The listing builds one solid part. Answer for the finished solid, in the listing's coordinates (mm). A direction names the side the tool comes from. Coordinates: 2 decimals unless noted, no trailing zeros. Loops run counter-clockwise (first coordinate to the right, second up) from the corner with the lowest first, then second, coordinate; pieces in that order, holes last. Notation, with made-up numbers: (78.25, 30) - (92.25, 30) arc R27 ccw to (92.25, 64) - close; hole circle Ø3 at (12, 0). An arc over 180 degrees is marked (long way). Return JSON: item names as keys, results as strings. Group by question number.
1. The mould has two halves that part along X. Classify faces 1 (the face through (-29.219, 17.594, 3.944)), 2 (the face through (11, 0, 8)): pulls with the +X half, pulls with the -X half, needs draft (parallel to the pull), parting line crosses it, or undercut.
2. Each of these flat-tipped pins is pushed along its axis until it touches: P1, Ø4, axis at y = -17.5, z = 4.5, coming from the -X side; P2, Ø4, axis at y = 19.5, z = 4, coming from the -X side; P3, Ø4, axis at x = 48, y = -18, coming from the +Z side; P4, Ø1.5, axis at x = 51, z = 1.5, coming from the +Y side. Where does it stop, or does it pass through?
3. Which of the six approach directions +Z, -Z, +X, -X, +Y, -Y give full straight-line access (tool end or side, diameter ignored) to faces 3 (the face through (40.757, 26.456, 3.944)), 4 (the face through (10, -29, 4))?
4. Find the intervals of material crossed by line 1 along Y through (x, z) = (10.75, 6); line 2 along X through (y, z) = (0.5, 2.5); line 3 along X through (y, z) = (-21.5, 1.25), in increasing order.
5. Section B-B (y = 1) is taken. Write down the section's boundary in (x, z), and give its area (3 significant figures).
6. Section A-A (x = -1) is taken. Write down the section's boundary in (y, z).
7. Section C-C (z = 3) is taken. State how many separate pieces and enclosed holes the cut face has, and give its area (3 significant figures).
8. Section D-D (x = 55) is taken. Write down the section's boundary in (y, z).
```python
from build123d import *

# Parameters (mm, degrees)
F0_R     = 1.6
F1_DEPTH = 8


with BuildPart() as f1:
    # F0 (on Top) → F1 (new body)
    with BuildSketch(Plane.XY):
        with BuildLine():
            ThreePointArc((7.75, 8.769357237), (9.5785114413, 4.5384947039), (10.2033247314, -0.028042301))
            ThreePointArc((10.2033247314, -0.028042301), (9.5785114413, -4.5945793059), (7.75, -8.825441839))
            Line((7.75, -8.825441839), (7.75, -18.0000000146))
            ThreePointArc((7.75, -18.0000000146), (10.7499999927, -15), (13.75, -18))
            Line((13.75, -18), (13.75, -8.8741196746))
            ThreePointArc((13.75, -8.8741196746), (11.25, 0), (13.75, 8.8741196746))
            Line((13.75, 8.8741196746), (13.75, 18))
            ThreePointArc((13.75, 18), (10.75, 15), (7.75, 18))
            Line((7.75, 18), (7.75, 8.769357237))
        make_face()
        with BuildLine():
            Line((7.75, 27.5), (7.75, 18))
            ThreePointArc((7.75, 18), (10.75, 21), (13.75, 18))
            Line((13.75, 18), (13.75, 27.5))
            Line((13.75, 27.5), (7.75, 27.5))
        make_face()
        with BuildLine():
            ThreePointArc((13.75, 18), (10.75, 21), (7.75, 18))
            ThreePointArc((7.75, 18), (10.75, 15), (13.75, 18))
        make_face()
        with Locations((10.75, 18)):
            Circle(F0_R, mode=Mode.SUBTRACT)
        with BuildLine():
            ThreePointArc((13.75, -18), (10.7499999927, -15), (7.75, -18.0000000146))
            ThreePointArc((7.75, -18.0000000146), (10.7500000073, -21), (13.75, -18))
        make_face()
        with Locations((10.75, -18)):
            Circle(F0_R, mode=Mode.SUBTRACT)
        with BuildLine():
            ThreePointArc((13.75, -18), (10.7500000073, -21), (7.75, -18.0000000146))
            Line((7.75, -18.0000000146), (7.75, -27.5))
            Line((7.75, -27.5), (13.75, -27.5))
            Line((13.75, -27.5), (13.75, -18))
        make_face()
        with BuildLine():
            ThreePointArc((-25.2919277241, 23.9346233209), (-18.7517090297, 26.593722392), (-11.75, 27.5))
            Line((-11.75, 27.5), (-11.75, 29))
            ThreePointArc((-11.75, 29), (-40.75, 0), (-11.75, -29))
            Line((-11.75, -29), (-11.75, -27.5))
            ThreePointArc((-11.75, -27.5), (-19.1538130954, -26.4845908341), (-26.0108698504, -23.5133492108))
            ThreePointArc((-26.0108698504, -23.5133492108), (-27.4397291664, -22.5850038451), (-28.8083510414, -21.5699480701))
            ThreePointArc((-28.8083510414, -21.5699480701), (-29.7732335043, -20.7704851664), (-30.7006958236, -19.9278982284))
            ThreePointArc((-30.7006958236, -19.9278982284), (-39.2465788178, -0.4337664292), (-31.3198462511, 19.3202256122))
            ThreePointArc((-31.3198462511, 19.3202256122), (-30.0815714824, 20.4988655048), (-28.77245464, 21.5982878495))
            ThreePointArc((-28.77245464, 21.5982878495), (-27.0767734107, 22.8328714098), (-25.2919277241, 23.9346233209))
        make_face()
        Polygon((-11.75, 29), (-11.75, 27.5), (7.75, 27.5), (13.75, 27.5), (33.25, 27.5), (33.25, 29), align=None)
        Polygon((7.75, -27.5), (-11.75, -27.5), (-11.75, -29), (33.25, -29), (33.25, -27.5), (13.75, -27.5), align=None)
        with BuildLine():
            Line((-23.9181566023, 16.8211807336), (-22.9196159905, 15.8385184773))
            ThreePointArc((-22.9196159905, 15.8385184773), (-22.2394609196, 16.8255111811), (-22, 18))
            ThreePointArc((-22, 18), (-22.2419209631, 19.180254221), (-22.9286666841, 20.1701562834))
            ThreePointArc((-22.9286666841, 20.1701562834), (-25.0876469222, 20.9987193962), (-27.1945482113, 20.0454725978))
            Line((-27.1945482113, 20.0454725978), (-26.1960075994, 19.0628103416))
            ThreePointArc((-26.1960075994, 19.0628103416), (-24.4314985308, 19.4955955601), (-23.4, 18))
            ThreePointArc((-23.4, 18), (-23.5352560913, 17.3561636218), (-23.9181566023, 16.8211807336))
        make_face()
        with BuildLine():
            ThreePointArc((-27.0590321397, 15.818168969), (-24.9852520778, 15.0000362504), (-22.9196159905, 15.8385184773))
            Line((-22.9196159905, 15.8385184773), (-23.9181566023, 16.8211807336))
            ThreePointArc((-23.9181566023, 16.8211807336), (-26.122267433, 16.8595984002), (-26.1960075994, 19.0628103416))
            Line((-26.1960075994, 19.0628103416), (-27.1945482113, 20.0454725978))
            ThreePointArc((-27.1945482113, 20.0454725978), (-27.9984596784, 17.9038773857), (-27.0590321397, 15.818168969))
        make_face()
        with BuildLine():
            Line((-22.9286666841, 20.1701562834), (-25.2919277241, 23.9346233209))
            ThreePointArc((-25.2919277241, 23.9346233209), (-27.0767734107, 22.8328714098), (-28.77245464, 21.5982878495))
            Line((-28.77245464, 21.5982878495), (-27.1945482113, 20.0454725978))
            ThreePointArc((-27.1945482113, 20.0454725978), (-25.0876469222, 20.9987193962), (-22.9286666841, 20.1701562834))
        make_face()
        with BuildLine():
            ThreePointArc((-22.3292838603, -18), (-22.5488627131, -16.9395045028), (-23.1714929463, -16.053390986))
            Line((-23.1714929463, -16.053390986), (-23.9378571629, -16.8033995681))
            ThreePointArc((-23.9378571629, -16.8033995681), (-23.5406459409, -17.3440383164), (-23.4, -18))
            ThreePointArc((-23.4, -18), (-24.4480811477, -19.5017941205), (-26.2192319756, -19.0360856093))
            Line((-26.2192319756, -19.0360856093), (-26.9855961921, -19.7860941914))
            ThreePointArc((-26.9855961921, -19.7860941914), (-24.9271170835, -20.6697214797), (-22.9199137797, -19.6751017924))
            ThreePointArc((-22.9199137797, -19.6751017924), (-22.4812657406, -18.8880892011), (-22.3292838603, -18))
        make_face()
        with BuildLine():
            Line((-23.9378571629, -16.8033995681), (-23.1714929463, -16.053390986))
            ThreePointArc((-23.1714929463, -16.053390986), (-25.0424895986, -15.3296218746), (-26.8895125058, -16.1125500829))
            ThreePointArc((-26.8895125058, -16.1125500829), (-27.6698030703, -17.9301697453), (-26.9855961921, -19.7860941914))
            Line((-26.9855961921, -19.7860941914), (-26.2192319756, -19.0360856093))
            ThreePointArc((-26.2192319756, -19.0360856093), (-26.1191027607, -16.8564926712), (-23.9378571629, -16.8033995681))
        make_face()
        with BuildLine():
            ThreePointArc((-28.8083510414, -21.5699480701), (-27.4397291664, -22.5850038451), (-26.0108698504, -23.5133492108))
            Line((-26.0108698504, -23.5133492108), (-22.9199137797, -19.6751017924))
            ThreePointArc((-22.9199137797, -19.6751017924), (-24.9271170835, -20.6697214797), (-26.9855961921, -19.7860941914))
            Line((-26.9855961921, -19.7860941914), (-28.8083510414, -21.5699480701))
        make_face()
        with BuildLine():
            Line((-31.3198462511, 19.3202256122), (-27.0590321397, 15.818168969))
            ThreePointArc((-27.0590321397, 15.818168969), (-27.9984596784, 17.9038773857), (-27.1945482113, 20.0454725978))
            Line((-27.1945482113, 20.0454725978), (-28.77245464, 21.5982878495))
            ThreePointArc((-28.77245464, 21.5982878495), (-30.0815714824, 20.4988655048), (-31.3198462511, 19.3202256122))
        make_face()
        with BuildLine():
            ThreePointArc((33.25, -29), (62.25, 0), (33.25, 29))
            Line((33.25, 29), (33.25, 27.5))
            ThreePointArc((33.25, 27.5), (40.8605006229, 26.4259395343), (47.8765184935, 23.2876567468))
            ThreePointArc((47.8765184935, 23.2876567468), (50.7935969105, 21.177162403), (53.4099454165, 18.7036520713))
            ThreePointArc((53.4099454165, 18.7036520713), (60.7498923776, 0.0769364868), (53.514283477, -18.5905571505))
            ThreePointArc((53.514283477, -18.5905571505), (51.1559396917, -20.8716871325), (48.5427019981, -22.8557053183))
            ThreePointArc((48.5427019981, -22.8557053183), (41.2411858865, -26.3133226356), (33.25, -27.5))
            Line((33.25, -27.5), (33.25, -29))
        make_face()
        with BuildLine():
            ThreePointArc((-26.9855961921, -19.7860941914), (-27.6698030703, -17.9301697453), (-26.8895125058, -16.1125500829))
            Line((-26.8895125058, -16.1125500829), (-30.7006958236, -19.9278982284))
            ThreePointArc((-30.7006958236, -19.9278982284), (-29.7732335043, -20.7704851664), (-28.8083510414, -21.5699480701))
            Line((-28.8083510414, -21.5699480701), (-26.9855961921, -19.7860941914))
        make_face()
        with BuildLine():
            ThreePointArc((53.4099454165, 18.7036520713), (50.7935969105, 21.177162403), (47.8765184935, 23.2876567468))
            Line((47.8765184935, 23.2876567468), (45.4902157392, 19.6434667518))
            ThreePointArc((45.4902157392, 19.6434667518), (48.8575101217, 20.8748350198), (51, 18))
            ThreePointArc((51, 18), (50.8256587545, 16.9922040865), (50.3228982644, 16.1015417695))
            Line((50.3228982644, 16.1015417695), (53.4099454165, 18.7036520713))
        make_face()
        with BuildLine():
            Line((46.1222517122, -20.3396712093), (48.5427019981, -22.8557053183))
            ThreePointArc((48.5427019981, -22.8557053183), (51.1559396917, -20.8716871325), (53.514283477, -18.5905571505))
            Line((53.514283477, -18.5905571505), (50.1028595569, -15.8603781447))
            ThreePointArc((50.1028595569, -15.8603781447), (50.7666386348, -16.8399523007), (51, -18))
            ThreePointArc((51, -18), (49.2974504107, -20.7049255871), (46.1222517122, -20.3396712093))
        make_face()
        with BuildLine():
            ThreePointArc((51, 18), (48.8575101217, 20.8748350198), (45.4902157392, 19.6434667518))
            ThreePointArc((45.4902157392, 19.6434667518), (45.3608334407, 16.5735358847), (48, 15))
            ThreePointArc((48, 15), (49.2854231421, 15.2893382089), (50.3228982644, 16.1015417695))
            ThreePointArc((50.3228982644, 16.1015417695), (50.8256587545, 16.9922040865), (51, 18))
        make_face()
        with BuildLine():
            ThreePointArc((49.6, 18), (49.1313708499, 16.8686291501), (48, 16.4))
            ThreePointArc((48, 16.4), (46.4, 18), (48, 19.6))
            ThreePointArc((48, 19.6), (49.1313708499, 19.1313708499), (49.6, 18))
        make_face(mode=Mode.SUBTRACT)
        with BuildLine():
            Line((45.5893930702, -19.7857699264), (46.1222517122, -20.3396712093))
            ThreePointArc((46.1222517122, -20.3396712093), (49.2974504107, -20.7049255871), (51, -18))
            ThreePointArc((51, -18), (50.7666386348, -16.8399523007), (50.1028595569, -15.8603781447))
            Line((50.1028595569, -15.8603781447), (49.6267696131, -15.4793610679))
            ThreePointArc((49.6267696131, -15.4793610679), (48.8479632079, -15.1223345576), (48, -15))
            ThreePointArc((48, -15), (45.3206988057, -16.6504278047), (45.5893930702, -19.7857699264))
        make_face()
        with BuildLine():
            ThreePointArc((49.6, -18), (46.8686291501, -19.1313708499), (48, -16.4))
            ThreePointArc((48, -16.4), (49.1313708499, -16.8686291501), (49.6, -18))
        make_face(mode=Mode.SUBTRACT)
    extrude(amount=F1_DEPTH)


solid = f1.part
```
The answers:
{
 "1": {"face 1": "undercut", "face 2": "needs draft"},
 "2": {"P1": "stops at x = -36.26", "P2": "stops at x = -34.87", "P3": "stops at z = 8", "P4": "stops at y = 23.49"},
 "3": {"face 3": "+Z, -Z", "face 4": "+Z, -Z, +X, -X, -Y"},
 "4": {"line 1": "y = -29 to -19.6, -16.4 to 16.4, 19.6 to 29", "line 2": "x = -40.75 to -39.25, 10.2 to 11.26, 60.75 to 62.25", "line 3": "x = -31.21 to -24.39, 7.75 to 13.75, 47.24 to 52.71"},
 "5": {"outline": "(-40.73, 0) - (-39.23, 0) - (-39.23, 8) - (-40.73, 8) - close; (10.17, 0) - (11.28, 0) - (11.28, 8) - (10.17, 8) - close; (60.73, 0) - (62.23, 0) - (62.23, 8) - (60.73, 8) - close", "area": "32.9 mm2"},
 "6": {"outline": "(-29, 0) - (-27.5, 0) - (-27.5, 8) - (-29, 8) - close; (27.5, 0) - (29, 0) - (29, 8) - (27.5, 8) - close"},
 "7": {"separate pieces": "1", "enclosed holes": "8", "area": "794 mm2"},
 "8": {"outline": "(-19.18, 0) - (-16.83, 0) - (-16.83, 8) - (-19.18, 8) - close; (16.83, 0) - (19.18, 0) - (19.18, 8) - (16.83, 8) - close"}
}
